Work out the finished part from the listing and answer in its coordinate system (mm). Round coordinates to 2 decimals unless told otherwise and drop trailing zeros. Loops run counter-clockwise (first coordinate to the right, second up) from the corner with the lowest first, then second, coordinate; pieces in that order, holes last. Notation, with made-up numbers: (69.25, -30.5) -> (74.25, -30.5) arc R14 cw to (74.25, -10.5) -> close; hole circle Ø3 at (-20, 24.25). An arc over 180 degrees is marked (long way). Use one line per item in the form item = value.
Autodesk Inventor part; units mm, degrees
ref_plane "YZ Plane" through (0, 0, 0) normal (1, 0, 0) x (0, 1, 0)
ref_plane "XZ Plane" through (0, 0, 0) normal (0, 1, 0) x (-1, 0, 0)
ref_plane "XY Plane" through (0, 0, 0) normal (0, 0, 1) x (1, 0, 0)
sketch "Sketch1" plane through (0, 0, 0) normal (0, 0, 1) x (1, 0, 0)
  line L0 (-546.1, -990.6) -> (546.1, -990.6)
  line L1 (546.1, -990.6) -> (546.1, 990.6)
  line L2 (546.1, 990.6) -> (-546.1, 990.6)
  line L3 (-546.1, 990.6) -> (-546.1, -990.6)
  line L4 (-546.1, -990.6) -> (546.1, 990.6) construction
  line L5 (546.1, -990.6) -> (-546.1, 990.6) construction
  point P0 (0, 0)
  dimension "d0" = 1092.2
  dimension "d1" = 1981.2
extrude "Extrusion1" add sketch "Sketch1" against normal blind 3.175
sketch "Sketch2" plane through (0, 0, 0) normal (0, 0, 1) x (1, 0, 0)
  line L0 (546.1, 990.6) -> (-546.1, 990.6)
  line L1 (-546.1, 990.6) -> (-546.1, -990.6)
  line L2 (-368.3, -508) -> (368.3, -508)
  line L3 (368.3, -508) -> (368.3, 101.6)
  line L4 (368.3, 101.6) -> (-368.3, 101.6)
  line L5 (-368.3, 101.6) -> (-368.3, -508)
  point P0 (0, 0)
  dimension "d4" = 736.6
  dimension "d6" = 609.6
  dimension "d7" = 889
  dimension "d8" = 177.8
extrude "Extrusion2" cut sketch "Sketch2" against normal up to next
properties part number "GE-13012B" material "Polyethylene, High Density"
(1) Consider L1, parallel to Y at x = -73.5, z = -1.25; L2, parallel to X at y = -363.5, z = -2.8. Determine where each line is inside the solid, lowest interval first.
Completed:
L1 = -990.6 to -508, 101.6 to 990.6
L2 = -546.1 to -368.3, 368.3 to 546.1
(2) Find section C-C, the plane y = -85. Write down the section's boundary in (x, z) (3 decimals).
Completed:
outline = (-546.1, -3.175) -> (-368.3, -3.175) -> (-368.3, 0) -> (-546.1, 0) -> close; (368.3, -3.175) -> (546.1, -3.175) -> (546.1, 0) -> (368.3, 0) -> close
(3) Given P1, Ø3, axis at x = -312.5, y = -561, coming from the +Z side, flat-ended and moving along its own axis, determine where the tip first touches the part or whether it passes through.
Completed:
P1 = 0
(4) Find section A-A, the plane z = -2.2. Write down the section's boundary in (x, y).
Completed:
outline = (-546.1, -990.6) -> (546.1, -990.6) -> (546.1, 990.6) -> (-546.1, 990.6) -> close; hole (-368.3, -508) -> (368.3, -508) -> (368.3, 101.6) -> (-368.3, 101.6) -> close
(5) Find section B-B, the plane x = 88. Write down the section's boundary in (y, z) (3 decimals), then the cut area to 3 significant figures.
Completed:
outline = (-990.6, -3.175) -> (-508, -3.175) -> (-508, 0) -> (-990.6, 0) -> close; (101.6, -3.175) -> (990.6, -3.175) -> (990.6, 0) -> (101.6, 0) -> close
area = 4,350 mm2
